Read the model definition and answer for the solid it produces. Units are mm, in the model's axes. Coordinates: 2 decimals unless noted, no trailing zeros. Loops run counter-clockwise (first coordinate to the right, second up) from the corner with the lowest first, then second, coordinate; pieces in that order, holes last.
from build123d import *

# Parameters (mm, degrees)
SKETCH1_R           = 24
BOSS_EXTRUDE1_DEPTH = 6.35


with BuildPart() as part:
    # Sketch1 → Boss-Extrude1 (new, symmetric)
    with BuildSketch(Plane(origin=(0, 0, 0), x_dir=(1, 0, 0), z_dir=(0, 1, 0))):
        with Locations(Location((0, 0, 0), (0, 0, 270))):
            Circle(SKETCH1_R)
        Polygon((-6.6, 18.75), (6.6, 18.75), (6.6, 13.25), (13.25, 13.25), (13.25, 6.6), (18.75, 6.6), (18.75, -6.6), (13.25, -6.6), (13.25, -13.25), (6.6, -13.25), (6.6, -18.75), (-6.6, -18.75), (-6.6, -13.25), (-13.25, -13.25), (-13.25, -6.6), (-18.75, -6.6), (-18.75, 6.6), (-13.25, 6.6), (-13.25, 13.25), (-6.6, 13.25), align=None, mode=Mode.SUBTRACT)
    extrude(amount=BOSS_EXTRUDE1_DEPTH, both=True)


solid = part.part
Q1. A cutting plane is placed at B-B (z = 0). Give the vertices of the cut face in (x, y).
Findings below:
outline: (-24, -6.35) - (-18.75, -6.35) - (-18.75, 6.35) - (-24, 6.35) - close; (18.75, -6.35) - (24, -6.35) - (24, 6.35) - (18.75, 6.35) - close
Q2. Flat-ended cylindrical pins translate along their axes: pin 1 Ø6 at (y, z) = (-4.5, 2.5) entering from -X; pin 2 Ø3.5 at (y, z) = (-1, 11) entering from -X; pin 3 Ø4.5 at (y, z) = (2, 15) entering from -X; pin 4 Ø6 at (x, z) = (-16, -6) entering from +Y. Find the tip coordinate at first contact, or state that the pin passes through.
Findings below:
pin 1: stops at x = -24
pin 2: stops at x = -22.15
pin 3: stops at x = -20.33
pin 4: stops at y = 6.35
Q3. Straight lines are drawn through the part: probe 1 along X at (y, z) = (-3, 0.5); probe 2 along X at (y, z) = (5, 13.5); probe 3 along Z at (x, y) = (-15.5, 0). For each, find the intervals that lie inside material, in ascending order.
Findings below:
probe 1: x = -23.99 to -18.75, 18.75 to 23.99
probe 2: x = -19.84 to -6.6, 6.6 to 19.84
probe 3: z = -18.32 to -6.6, 6.6 to 18.32
Q4. A cutting plane is placed at A-A (x = 0). Give the vertices of the cut face in (y, z).
Findings below:
outline: (-6.35, -24) - (6.35, -24) - (6.35, -18.75) - (-6.35, -18.75) - close; (-6.35, 18.75) - (6.35, 18.75) - (6.35, 24) - (-6.35, 24) - close
Q5. A cutting plane is placed at C-C (y = -0.25). Give the vertices of the cut face in (x, z), then the cut area to 3 significant figures.
Findings below:
outline: circle Ø48 at (0, 0); hole (-18.75, -6.6) - (-13.25, -6.6) - (-13.25, -13.25) - (-6.6, -13.25) - (-6.6, -18.75) - (6.6, -18.75) - (6.6, -13.25) - (13.25, -13.25) - (13.25, -6.6) - (18.75, -6.6) - (18.75, 6.6) - (13.25, 6.6) - (13.25, 13.25) - (6.6, 13.25) - (6.6, 18.75) - (-6.6, 18.75) - (-6.6, 13.25) - (-13.25, 13.25) - (-13.25, 6.6) - (-18.75, 6.6) - close
area: 817 mm2
Q6. Determine the mould class of faces 1 (the face through (-18.75, 0, 0)), 2 (the face through (14, 6.35, 7)), 3 (the face through (10, 0, 13.25)), 4 (the face through (7.21, 0.09, 22.89)) for opening direction Z: +Z half, -Z half, draft (parallel to the pull), parting line (faces both ways), or undercut.
Findings below:
face 1: undercut
face 2: draft
face 3: undercut
face 4: parting line
